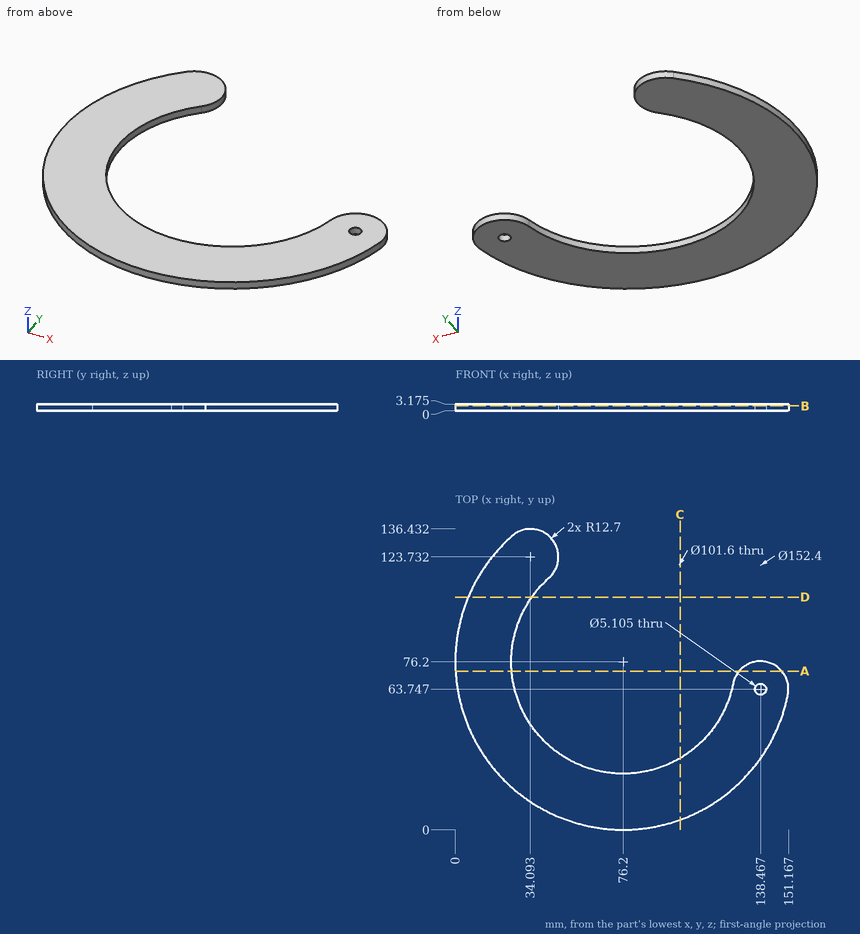
Answer from the drawing. Dimensions are ordinates in mm from the lowest x, y and z of the part. Give positions to 0.01 mm unless a question says otherwise; leave off trailing zeros. Write each loop counter-clockwise with the first axis right and the second up, starting at its lowest first coordinate (ties: lowest second). Pieces come first, ordered by that corner, then holes. Notation, with made-up numbers: M -26.75,35 L -15.75,35 A22 ccw -15.75,74 Z; hole C -21.75,60.25 d11. An arc over 180 degrees is marked long. Answer as CSV lines item,"result".
Q1. Given P1, Ø6, axis at x = 138.47, y = 63.75, coming from the +Z side (3 decimals); P2, Ø1, axis at x = 39, z = 1, coming from the -Y side; P3, Ø1, axis at y = 116, z = 1, coming from the -X side, each flat-ended and moving along its own axis, determine where each tip first touches the part or whether it passes through.
A:
P1,"stops at z = 3.175"
P2,"stops at y = 9.42"
P3,"stops at x = 10.92"
Q2. A cutting plane is placed at B-B on z = 2.3. Write down the section's boundary in (x, y) (1 decimal).
A:
outline,"M 25.7,133.2 A76.2 ccw long 150.9,61.3 A12.7 ccw 126,66.2 A50.8 cw long 42.5,114.2 A12.7 ccw Z; hole C 138.5,63.7 d5.1"
Q3. A cutting plane is placed at A-A on y = 72. Write down the section's boundary in (x, z) (1 decimal), plus the area to 3 significant figures.
A:
outline,"M 0.1,0 L 25.6,0 L 25.6,3.2 L 0.1,3.2 Z; M 128.8,0 L 148.1,0 L 148.1,3.2 L 128.8,3.2 Z"
area,"142 mm²"
Q4. A cutting plane is placed at D-D on y = 105.5. Write down the section's boundary in (x, z) (1 decimal).
A:
outline,"M 5.9,0 L 34.7,0 L 34.7,3.2 L 5.9,3.2 Z"
Q5. Find the intervals of material crossed by probe 1 along X at (y, z) = (65.5, 0.65) (1 decimal); probe 2 along Y at (x, z) = (76.2, 1.85); probe 3 along X at (y, z) = (45.5, 2.75) (1 decimal), in increasing order. Write a range as [from, to].
A:
probe 1,"x = [0.8, 26.5], [125.9, 136.6], [140.3, 151]"
probe 2,"y = [0, 25.4]"
probe 3,"x = [6.5, 35.7], [116.7, 145.9]"
Q6. A cutting plane is placed at C-C on x = 102. Write down the section's boundary in (y, z) (1 decimal).
A:
outline,"M 4.5,0 L 32.4,0 L 32.4,3.2 L 4.5,3.2 Z"
